For this review, take the finished solid that the model builds, in its own axes (mm). Round coordinates to 2 decimals unless told otherwise and drop trailing zeros. Order: outer loops, then holes, each group sorted by start corner. A loop starts at its lowest first (then second) coordinate and runs counter-clockwise, first axis right, second up. Notation, with made-up numbers: (-7, -5) - (47, -5) arc R28 cw to (47, 17) - close; hole circle Ø7 at (29, 73). An arc over 180 degrees is marked (long way). One line per item, written item: value.
```python
from build123d import *
from OCP.BRepFilletAPI import BRepFilletAPI_MakeFillet

# Parameters (mm, degrees)
SKETCH1_R           = 2.5
BOSS_EXTRUDE1_DEPTH = 3
BOSS_EXTRUDE3_DEPTH = 3
FILLET1_R1          = 5
FILLET1_R2          = 15
FILLET1_R3          = 20
FILLET1_R4          = 2
SKETCH3_6_R         = 1.5
CUT_EXTRUDE2_DEPTH  = 62.394217969


with BuildPart() as part:
    # Sketch1 → Boss-Extrude1 (new body)
    with BuildSketch(Plane.XY):
        Polygon((-32.5, 30), (32.5, 30), (32.5, -10), (0, -35), (-32.5, -10), align=None)
        with Locations((25, 20)):
            Circle(SKETCH1_R, mode=Mode.SUBTRACT)
        with Locations((-25, 20)):
            Circle(SKETCH1_R, mode=Mode.SUBTRACT)
        with BuildLine():
            Line((2.5, -16.5), (2.5, -23.5))
            ThreePointArc((2.5, -23.5), (0, -26), (-2.5, -23.5))
            Line((-2.5, -23.5), (-2.5, -16.5))
            ThreePointArc((-2.5, -16.5), (0, -14), (2.5, -16.5))
        make_face(mode=Mode.SUBTRACT)
    extrude(amount=BOSS_EXTRUDE1_DEPTH)

    # Sketch3 → Boss-Extrude3 (add)
    with BuildSketch(Plane.XY.offset(3)):
        with BuildLine():
            ThreePointArc((-15.5, 44), (-16.560660172, 46.560660172), (-14, 45.5))
            Line((-14, 45.5), (14, 45.5))
            ThreePointArc((14, 45.5), (15.5, 47), (17, 45.5))
            ThreePointArc((17, 45.5), (16.560660172, 44.439339828), (15.5, 44))
            Line((15.5, 44), (15.5, 30))
            Line((15.5, 30), (21.5, 30))
            Line((21.5, 30), (21.5, 52))
            Line((21.5, 52), (-21.5, 52))
            Line((-21.5, 52), (-21.5, 30))
            Line((-21.5, 30), (-15.5, 30))
            Line((-15.5, 30), (-15.5, 44))
        make_face()
        with BuildLine():
            Line((14, 45.5), (-14, 45.5))
            ThreePointArc((-14, 45.5), (-14.439339828, 44.439339828), (-15.5, 44))
            Line((-15.5, 44), (-15.5, 30))
            Line((-15.5, 30), (-11, 30))
            ThreePointArc((-11, 30), (0, 41), (11, 30))
            Line((11, 30), (15.5, 30))
            Line((15.5, 30), (15.5, 44))
            ThreePointArc((15.5, 44), (14.439339828, 44.439339828), (14, 45.5))
        make_face()
    extrude(amount=-BOSS_EXTRUDE3_DEPTH)

    # Fillet1: one fillet with a radius per group of edges: ONE call of the kernel's fillet builder (fillet() takes one radius for all edges)
    fillet1_edges_1 = [part.edges().sort_by_distance(p)[0] for p in [
        (32.5, 30, 1.5),
        (-32.5, 30, 1.5),
        (-21.5, 52, 1.5),
        (21.5, 52, 1.5),
    ]]
    fillet1_edges_2 = [part.edges().sort_by_distance(p)[0] for p in [
        (-32.5, -10, 1.5),
        (32.5, -10, 1.5),
    ]]
    fillet1_edges_3 = [part.edges().sort_by_distance(p)[0] for p in [
        (0, -35, 1.5),
    ]]
    fillet1_edges_4 = [part.edges().sort_by_distance(p)[0] for p in [
        (21.5, 30, 1.5),
        (-21.5, 30, 1.5),
    ]]
    fillet1 = BRepFilletAPI_MakeFillet(part.part.solid().wrapped)
    for e in fillet1_edges_1:
        fillet1.Add(FILLET1_R1, e.wrapped)
    for e in fillet1_edges_2:
        fillet1.Add(FILLET1_R2, e.wrapped)
    for e in fillet1_edges_3:
        fillet1.Add(FILLET1_R3, e.wrapped)
    for e in fillet1_edges_4:
        fillet1.Add(FILLET1_R4, e.wrapped)
    add(Compound.cast(fillet1.Shape()), mode=Mode.REPLACE)

    # Sketch3<6> → Cut-Extrude2 (cut, through all)
    with BuildSketch(Plane.XY.offset(3)):
        with Locations((15.5, 14.5)):
            Circle(SKETCH3_6_R)
        with Locations((-15.5, 14.5)):
            Circle(SKETCH3_6_R)
        with BuildLine():
            ThreePointArc((-11, 30), (0, 19), (11, 30))
            Line((11, 30), (-11, 30))
        make_face()
        with BuildLine():
            Line((-11, 30), (11, 30))
            ThreePointArc((11, 30), (0, 41), (-11, 30))
        make_face()
    extrude(amount=-CUT_EXTRUDE2_DEPTH, mode=Mode.SUBTRACT)


solid = part.part
```
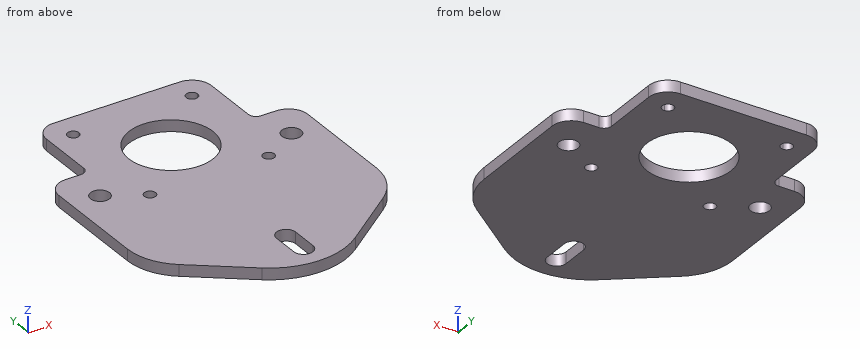
Item 1: Take a section at B-B (y = 14.5). Write out the cut boundary in (x, z), plus the area to 3 significant figures.
Returned:
outline: (-32.5, 0) - (-17, 0) - (-17, 3) - (-32.5, 3) - close; (-14, 0) - (14, 0) - (14, 3) - (-14, 3) - close; (17, 0) - (32.5, 0) - (32.5, 3) - (17, 3) - close
area: 177 mm^2
Item 2: Take a section at C-C (z = 1.25). Count the separate pieces of the cut face and the enclosed holes in it, plus the area to 3 significant figures.
Returned:
separate pieces: 1
enclosed holes: 8
area: 3,780 mm^2
Item 3: Wall thickness on line 1 (Y direction, x = -15.5, z = 0.95); line 2 (X direction, y = -17, z = 0.65); line 3 (X direction, y = 32, z = 0.85): over which ranges is each line inside the solid? List them lowest first.
Returned:
line 1: -23.08 to 13, 16 to 44, 47 to 52
line 2: -23.4 to -2.5, 2.5 to 23.4
line 3: -21.5 to -10.82, 10.82 to 21.5
Item 4: For P1, Ø20, axis at x = 0, y = 30, coming from the +Z side; P2, Ø3.5, axis at x = 15.5, y = 14.5, coming from the +Z side; P3, Ø0.9, axis at y = 42, z = 2, coming from the +X side; P4, Ø1.5, axis at y = -18.5, z = 1.5, coming from the +X side (3 decimals), all flat-tipped, find the tip position at first contact; note any pin that passes through.
Returned:
P1: through
P2: z = 3
P3: x = 21.5
P4: x = 22.425
Item 5: Take a section at A-A (x = 0). Write out the cut boundary in (y, z).
Returned:
outline: (-29.77, 0) - (-26, 0) - (-26, 3) - (-29.77, 3) - close; (-14, 0) - (19, 0) - (19, 3) - (-14, 3) - close; (41, 0) - (52, 0) - (52, 3) - (41, 3) - close
Item 6: Take a section at D-D (x = 8.5). Write out the cut boundary in (y, z).
Returned:
outline: (-27.87, 0) - (23.02, 0) - (23.02, 3) - (-27.87, 3) - close; (36.98, 0) - (52, 0) - (52, 3) - (36.98, 3) - close
